Read the model definition and answer for the solid it produces. Units are mm, in the model's axes. A direction names the side the tool comes from. Coordinates: 2 decimals unless noted, no trailing zeros. Write each loop counter-clockwise with the first axis right and the second up, starting at its lowest first coordinate (ties: lowest second). Pieces come first, ordered by that corner, then holes. Notation, with made-up numbers: M 26.25,72 L 52.25,72 A6 ccw 52.25,78 Z; hole C 79,12.25 d4. An arc over 180 degrees is marked long. Write item = value, one per line.
from build123d import *

# Parameters (mm, degrees)
F0_W     = 40
F0_H     = 80
F1_DEPTH = 30
F2_R     = 5
F4_DEPTH = 30
F5_R     = 5
F6_DEPTH = 40.001


with BuildPart() as f1:
    # F0 (on Top) → F1 (new body)
    with BuildSketch(Plane.XY):
        Rectangle(F0_W, F0_H)
    extrude(amount=F1_DEPTH)

    # F2
    f2_edges = [f1.edges().sort_by_distance(p)[0] for p in [
        (20, 40, 15),
        (-20, 40, 15),
        (-20, -40, 15),
        (20, -40, 15),
    ]]
    fillet(f2_edges, radius=F2_R)

    # F3 (on face) → F4 (cut)
    with BuildSketch(Plane.XY.offset(30)):
        with BuildLine():
            ThreePointArc((17, 35), (16.414214, 36.414214), (15, 37))
            Line((15, 37), (-15, 37))
            ThreePointArc((-15, 37), (-16.414214, 36.414214), (-17, 35))
            Line((-17, 35), (-17, -35))
            ThreePointArc((-17, -35), (-16.414214, -36.414214), (-15, -37))
            Line((-15, -37), (15, -37))
            ThreePointArc((15, -37), (16.414214, -36.414214), (17, -35))
            Line((17, -35), (17, 35))
        make_face()
    extrude(amount=-F4_DEPTH, mode=Mode.SUBTRACT)

    # F5 (on face) → F6 (cut, through all)
    with BuildSketch(Plane.YZ.offset(20)):
        with Locations((0, 15)):
            Circle(F5_R)
    extrude(amount=-F6_DEPTH, mode=Mode.SUBTRACT)


solid = f1.part
Item 1: Consider line 1 along X through (y, z) = (16.5, 18); line 2 along Y through (x, z) = (1.5, 19.5); line 3 along Z through (x, y) = (18.05, 0). Determine where each line is inside the solid, lowest interval first. Write a range as from..to.
Worked answers:
line_1 = -20..-17, 17..20
line_2 = -40..-37, 37..40
line_3 = 0..10, 20..30
Item 2: Find section A-A (y = 28.5). Determine the outline of the cut face in (x, z), and give its area (3 significant figures).
Worked answers:
outline = M -20,0 L -17,0 L -17,30 L -20,30 Z; M 17,0 L 20,0 L 20,30 L 17,30 Z
area = 180 mm²
Item 3: Find section B-B (z = 15). Determine the outline of the cut face in (x, y), and give its area (3 significant figures).
Worked answers:
outline = M -20,-35 A5 ccw -15,-40 L 15,-40 A5 ccw 20,-35 L 20,-5 L 17,-5 L 17,-35 A2 cw 15,-37 L -15,-37 A2 cw -17,-35 L -17,-5 L -20,-5 Z; M -20,5 L -17,5 L -17,35 A2 cw -15,37 L 15,37 A2 cw 17,35 L 17,5 L 20,5 L 20,35 A5 ccw 15,40 L -15,40 A5 ccw -20,35 Z
area = 606 mm²
Item 4: Find section D-D (y = 0). Determine the outline of the cut face in (x, z).
Worked answers:
outline = M -20,0 L -17,0 L -17,10 L -20,10 Z; M -20,20 L -17,20 L -17,30 L -20,30 Z; M 17,0 L 20,0 L 20,10 L 17,10 Z; M 17,20 L 20,20 L 20,30 L 17,30 Z
Item 5: Which of the six approach directions +Z, -Z, +X, -X, +Y, -Y give full straight-line access (tool end or side, diameter ignored) to faces 5 (the face through (19, 38, 15)), 6 (the face through (16.43, 36.4, 15.21))?
Worked answers:
face_5 = +Z, -Z, +X, +Y
face_6 = +Z, -Z
Item 6: A flat-ended cylindrical pin translates along its axis: pin 1 (9 mm diameter, centred on y = 0, z = 15, fed in from -X). Find the tip coordinate at first contact, or state that the pin passes through.
Worked answers:
pin_1 = through
Item 7: Find section C-C (x = -14). Determine the outline of the cut face in (y, z).
Worked answers:
outline = M -40,0 L -37,0 L -37,30 L -40,30 Z; M 37,0 L 40,0 L 40,30 L 37,30 Z
Item 8: For a pull along Z with two mould halves and no side action, classify faces 1 (the face through (-18, 0, 30)), 2 (the face through (-18, 0, 0)), 3 (the face through (-18.48, -1.08, 10.12)), 4 (the face through (0, -40, 15)) as released by +Z, released by -Z, zero draft, split by the parting line, or undercut.
Worked answers:
face_1 = released by +Z
face_2 = released by -Z
face_3 = undercut
face_4 = zero draft
